from build123d import *

# Parameters (mm, degrees)
SKETCH3_R               = 11.5
SKETCH3_R_2             = 1.75
BOSS_EXTRUDE1_DEPTH     = 19
CUT_EXTRUDE1_START      = 19
SKETCH3_3_R             = 11.5
SKETCH3_3_R_2           = 1.75
CUT_EXTRUDE1_DEPTH      = 17
SKETCH3_4_R             = 1.75
SKETCH3_4_R_2           = 11.5
CUT_EXTRUDE3_DEPTH      = 38.975320933
CUT_EXTRUDE7_DEPTH      = 38.975320933
CUT_EXTRUDE7_DEPTH_BACK = 38.975320933
CUT_EXTRUDE8_DEPTH      = 38.015199581
BOSS_EXTRUDE4_DEPTH     = 19
BOSS_EXTRUDE5_START     = 19
BOSS_EXTRUDE5_DEPTH     = 3
BOSS_EXTRUDE6_DEPTH     = 6
BOSS_EXTRUDE7_START     = -6
BOSS_EXTRUDE7_DEPTH     = 16
SKETCH14_R              = 7
BOSS_EXTRUDE8_DEPTH     = 3
SKETCH15_R              = 3
CUT_EXTRUDE10_DEPTH     = 13


# Read off the part's stored shape, not the designer's step: Boss-Extrude7
with BuildPart() as part:
    # Sketch3 → Boss-Extrude1 (new body)
    # profile 1 of 7: a face of its own
    with BuildSketch(Plane.XY):
        Polygon((-23.25, 17.798989873), (-17.798989873, 23.25), (17.798989873, 23.25), (23.25, 17.798989873), (23.25, -17.798989873), (17.798989873, -23.25), (-17.798989873, -23.25), (-23.25, -17.798989873), align=None)
        Polygon((21.25, 16.970562748), (16.970562748, 21.25), (-16.970562748, 21.25), (-21.25, 16.970562748), (-21.25, -16.970562748), (-16.970562748, -21.25), (16.970562748, -21.25), (21.25, -16.970562748), align=None, mode=Mode.SUBTRACT)
    # profile 2 of 7: a face of its own
    with BuildSketch(Plane.XY):
        Polygon((21.25, 16.970562748), (21.25, -16.970562748), (16.970562748, -21.25), (-16.970562748, -21.25), (-21.25, -16.970562748), (-21.25, 16.970562748), (-16.970562748, 21.25), (16.970562748, 21.25), align=None)
        Circle(SKETCH3_R, mode=Mode.SUBTRACT)
        with Locations((-15.5, -15.5)):
            Circle(SKETCH3_R_2, mode=Mode.SUBTRACT)
        with Locations((15.5, -15.5)):
            Circle(SKETCH3_R_2, mode=Mode.SUBTRACT)
        with Locations((15.5, 15.5)):
            Circle(SKETCH3_R_2, mode=Mode.SUBTRACT)
        with Locations((-15.5, 15.5)):
            Circle(SKETCH3_R_2, mode=Mode.SUBTRACT)
    # profile 3 of 7: a face of its own
    with BuildSketch(Plane.XY):
        with Locations((-15.5, 15.5)):
            Circle(SKETCH3_R_2)
    # profile 4 of 7: a face of its own
    with BuildSketch(Plane.XY):
        with Locations((15.5, 15.5)):
            Circle(SKETCH3_R_2)
    # profile 5 of 7: a face of its own
    with BuildSketch(Plane.XY):
        with Locations((15.5, -15.5)):
            Circle(SKETCH3_R_2)
    # profile 6 of 7: a face of its own
    with BuildSketch(Plane.XY):
        with Locations((-15.5, -15.5)):
            Circle(SKETCH3_R_2)
    # profile 7 of 7: a face of its own
    with BuildSketch(Plane.XY):
        Circle(SKETCH3_R)
    extrude(amount=BOSS_EXTRUDE1_DEPTH)

    # Sketch3<3> → Cut-Extrude1 (cut)
    with BuildSketch(Plane.XY.offset(CUT_EXTRUDE1_START)):
        Polygon((21.25, 16.970562748), (21.25, -16.970562748), (16.970562748, -21.25), (-16.970562748, -21.25), (-21.25, -16.970562748), (-21.25, 16.970562748), (-16.970562748, 21.25), (16.970562748, 21.25), align=None)
        Circle(SKETCH3_3_R, mode=Mode.SUBTRACT)
        with Locations((-15.5, -15.5)):
            Circle(SKETCH3_3_R_2, mode=Mode.SUBTRACT)
        with Locations((15.5, -15.5)):
            Circle(SKETCH3_3_R_2, mode=Mode.SUBTRACT)
        with Locations((15.5, 15.5)):
            Circle(SKETCH3_3_R_2, mode=Mode.SUBTRACT)
        with Locations((-15.5, 15.5)):
            Circle(SKETCH3_3_R_2, mode=Mode.SUBTRACT)
    extrude(amount=-CUT_EXTRUDE1_DEPTH, mode=Mode.SUBTRACT)

    # Sketch3<4> → Cut-Extrude3 (cut, through all)
    with BuildSketch(Plane.XY):
        with Locations(Location((-15.5, 15.5, 0), (0, 0, 180))):
            Circle(SKETCH3_4_R)
        with Locations(Location((15.5, 15.5, 0), (0, 0, 180))):
            Circle(SKETCH3_4_R)
        with Locations(Location((-15.5, -15.5, 0), (0, 0, 180))):
            Circle(SKETCH3_4_R)
        with Locations(Location((0, 0, 0), (0, 0, 180))):
            Circle(SKETCH3_4_R_2)
        with Locations(Location((15.5, -15.5, 0), (0, 0, 180))):
            Circle(SKETCH3_4_R)
    extrude(amount=CUT_EXTRUDE3_DEPTH, mode=Mode.SUBTRACT)

    # Sketch6 → Cut-Extrude7 (cut, two sides: drawn at the far end of the back side and taken through both)
    with BuildSketch(Plane(origin=(0, 0, 0), x_dir=(0, 0, -1), z_dir=(1, 0, 0)).offset(-CUT_EXTRUDE7_DEPTH_BACK)):
        Polygon((-19, 23.25), (-5, 23.25), (-19, -17.798989873), align=None)
    extrude(amount=CUT_EXTRUDE7_DEPTH + CUT_EXTRUDE7_DEPTH_BACK, mode=Mode.SUBTRACT)

    # Sketch8 → Cut-Extrude8 (cut, through all)
    with BuildSketch(Plane.XY.offset(2)):
        Polygon((-16.970562748, 21.25), (-14.970562748, 23.25), (14.970562748, 23.25), (16.970562748, 21.25), align=None)
    extrude(amount=CUT_EXTRUDE8_DEPTH, mode=Mode.SUBTRACT)

    # Sketch10 → Boss-Extrude4 (add)
    with BuildSketch(Plane.XY):
        Polygon((19.798989873, -21.25), (-19.798989873, -21.25), (-15.048989873, -26), (15.048989873, -26), align=None)
    extrude(amount=BOSS_EXTRUDE4_DEPTH)

    # Sketch11 → Boss-Extrude5 (add)
    with BuildSketch(Plane.XY.offset(BOSS_EXTRUDE5_START)):
        with BuildLine():
            Line((-14.556349186, -21.25), (14.556349186, -21.25))
            ThreePointArc((14.556349186, -21.25), (15.480228719, -21.867316568), (15.263455967, -22.957106781))
            Line((15.263455967, -22.957106781), (12.220562748, -26))
            Line((12.220562748, -26), (-12.220562748, -26))
            Line((-12.220562748, -26), (-15.263455967, -22.957106781))
            ThreePointArc((-15.263455967, -22.957106781), (-15.480228719, -21.867316568), (-14.556349186, -21.25))
        make_face()
    extrude(amount=BOSS_EXTRUDE5_DEPTH)


with BuildPart() as body_2:
    # Sketch12 → Boss-Extrude6 (new body)
    with BuildSketch(Plane.XY):
        with BuildLine():
            Line((2.5, -28.5), (2.5, -49.75))
            ThreePointArc((2.5, -49.75), (1.767766953, -51.517766953), (0, -52.25))
            Line((0, -52.25), (0, -57.25))
            Line((0, -57.25), (10.5, -57.25))
            Line((10.5, -57.25), (10.5, -30.548989873))
            Line((10.5, -30.548989873), (15.048989873, -26))
            Line((15.048989873, -26), (0, -26))
            ThreePointArc((0, -26), (1.767766953, -26.732233047), (2.5, -28.5))
        make_face()
    extrude(amount=BOSS_EXTRUDE6_DEPTH)

    # Boss-Extrude7 outline → Boss-Extrude7 (add)
    with BuildSketch(Plane.XY.offset(6).offset(BOSS_EXTRUDE7_START)):
        with BuildLine():
            Line((7.5, -26), (0, -26))
            ThreePointArc((0, -26), (1.767766953, -26.732233047), (2.5, -28.5))
            Line((2.5, -28.5), (2.5, -49.75))
            ThreePointArc((2.5, -49.75), (1.767766953, -51.517766953), (0, -52.25))
            Line((0, -52.25), (0, -57.25))
            Line((0, -57.25), (3.562803405, -57.25))
            ThreePointArc((3.562803405, -57.25), (6.143187845, -60.341660723), (10, -61.5))
            Line((10, -61.5), (15, -61.5))
            Line((15, -61.5), (15, -64.75))
            Line((15, -64.75), (30, -64.75))
            Line((30, -64.75), (30, -61.75))
            Line((30, -61.75), (16.619881116, -56.775340415))
            ThreePointArc((16.619881116, -56.775340415), (14.864528014, -49.466475668), (7.5, -47.961651585))
            Line((7.5, -47.961651585), (7.5, -26))
        make_face()
    extrude(amount=BOSS_EXTRUDE7_DEPTH)

    # Sketch14 → Boss-Extrude8 (add)
    with BuildSketch(Plane.XY.offset(16)):
        with Locations((10, -54.5)):
            Circle(SKETCH14_R)
    extrude(amount=BOSS_EXTRUDE8_DEPTH)

    # Sketch15 → Cut-Extrude10 (cut)
    with BuildSketch(Plane.XY):
        with Locations((10, -54.5)):
            Circle(SKETCH15_R)
        with BuildLine():
            Line((16.866218411, -56.866927358), (17.214706637, -55.9296142))
            Line((17.214706637, -55.9296142), (12.996797424, -54.361417185))
            ThreePointArc((12.996797424, -54.361417185), (12.999199249, -54.430690092), (13, -54.5))
            ThreePointArc((13, -54.5), (12.966794868, -54.94511595), (12.867914527, -55.380378478))
            Line((12.867914527, -55.380378478), (16.866218411, -56.866927358))
        make_face()
    extrude(amount=CUT_EXTRUDE10_DEPTH, mode=Mode.SUBTRACT)


with BuildPart() as body_3:
    # Mirror1: mirrored copy
    add(body_2.part.mirror(Plane(origin=(0, 0, 0), x_dir=(0, 0, 1), z_dir=(1, 0, 0))))


with BuildPart() as body_2_1:
    add(body_2.part)

    # Combine1: union body 3, part
    add(body_3.part)
    add(part.part)


solid = body_2_1.part
Geometry: final body of the model. Coordinates: model frame, mm. A direction names the side the tool comes from. Coordinates: 2 decimals unless noted, no trailing zeros. Loops run counter-clockwise (first coordinate to the right, second up) from the corner with the lowest first, then second, coordinate; pieces in that order, holes last. Notation, with made-up numbers: (-29.75, -39) - (9.25, -39) arc R14 ccw to (9.25, -31) - close; hole circle Ø1 at (-8, -22). An arc over 180 degrees is marked (long way). One line per question, with ' | ' between items. Start each with the question number.
(1) Draft query along X for faces 5 (the flat face through (-23.25, -4, 7)), 6 (the flat face through (-18, -22, 19)), 7 (the flat face through (0, -21.25, 12)). Return one class per face: +X half, -X half, draft (parallel to the pull), parting line (faces both ways), or undercut.
(2) Cut plane B-B on x = 8.5. Output: boundary loops of the cut face in (y, z), and give its area (3 significant figures).
(3) Ray query, L1, parallel to X at y = 15.5, z = 1.35; L2, parallel to X at y = -11.5, z = 11; L3, parallel to Z at x = 17.5, y = -20. Return the intervals inside material, ascending. Write a range as from..to.
(4) Cut plane C-C on y = -10. Output: boundary loops of the cut face in (x, z).
(5) Cut plane A-A on y = 15.5. Output: boundary loops of the cut face in (x, z).
(6) Cut plane D-D on y = -42. Output: boundary loops of the cut face in (x, z).
(7) Reachability of faces 1 (the flat face through (-14.96, -55.09, 6.41)), 2 (the flat face through (-18.15, 20.07, 3.96)), 3 (the flat face through (2.5, -39, 8)), 4 (the cylindrical face through (-15.486, -21.883, 20.479)) from +Z, -Z, +X, -X, +Y, -Y: full face, straight path, thin tool, end or side. Return the list, or none.
(8) First-contact query: pin 1 (3 mm diameter, centred on x = -4.5, z = 8.5, fed in from +Y); pin 2 (8.5 mm diameter, centred on y = 3, z = 14.5, fed in from -X); pin 3 (10 mm diameter, centred on y = -45, z = 18, fed in from -X); pin 4 (8 mm diameter, centred on x = -2, y = 3, fed in from -Z). Flat tips, straight axial feed; report the tip coordinate or a pass-through.
Here are the results:
1) face 5: -X half | face 6: draft | face 7: undercut
2) outline: (-61.34, 0) - (-57.1, 0) - (-57.1, 13) - (-51.9, 13) - (-51.9, 0) - (-7.75, 0) - (-7.75, 2) - (-21.25, 2) - (-21.25, 22) - (-26, 22) - (-26, 6) - (-47.66, 6) - (-47.66, 19) - (-61.34, 19) - close; (7.75, 0) - (23.25, 0) - (23.25, 2) - (7.75, 2) - close | area: 485 mm²
3) L1: -23.25..-17.25, -13.75..13.75, 17.25..23.25 | L2: -23.25..-21.25, 21.25..23.25 | L3: 0..2
4) outline: (-23.25, 0) - (-5.68, 0) - (-5.68, 2) - (-21.25, 2) - (-21.25, 16.34) - (-23.25, 16.34) - close; (5.68, 0) - (23.25, 0) - (23.25, 16.34) - (21.25, 16.34) - (21.25, 2) - (5.68, 2) - close
5) outline: (-23.25, 0) - (-17.25, 0) - (-17.25, 2) - (-21.25, 2) - (-21.25, 7.64) - (-23.25, 7.64) - close; (-13.75, 0) - (13.75, 0) - (13.75, 2) - (-13.75, 2) - close; (17.25, 0) - (23.25, 0) - (23.25, 7.64) - (21.25, 7.64) - (21.25, 2) - (17.25, 2) - close
6) outline: (-10.5, 0) - (-2.5, 0) - (-2.5, 16) - (-7.5, 16) - (-7.5, 6) - (-10.5, 6) - close; (2.5, 0) - (10.5, 0) - (10.5, 6) - (7.5, 6) - (7.5, 16) - (2.5, 16) - close
7) face 1: -Z | face 2: +Z | face 3: +Z, -Z | face 4: +Z, -X
8) pin 1: y = -21.25 | pin 2: x = -23.25 | pin 3: x = -15.36 | pin 4: through
